from build123d import *

# Parameters (mm, degrees)
REVOLVE1_ANGLE = 270


with BuildPart() as part:
    # Sketch1 → Revolve1 (revolve)
    with BuildSketch(Plane.XY):
        with BuildLine():
            Line((0, 167.582815348), (0, 163))
            ThreePointArc((0, 163), (21.692969078, 161.550038974), (43, 157.225952056))
            Line((43, 157.225952056), (43, 87.225952056))
            Line((43, 87.225952056), (50, 87.225952056))
            Line((50, 87.225952056), (50, 57.225952056))
            Line((50, 57.225952056), (58, 57.225952056))
            Line((58, 57.225952056), (58, 112.225952056))
            Line((58, 112.225952056), (53, 112.225952056))
            Line((53, 112.225952056), (53, 117.225952056))
            Line((53, 117.225952056), (58, 117.225952056))
            Line((58, 117.225952056), (58, 122.225952056))
            Line((58, 122.225952056), (53, 122.225952056))
            Line((53, 122.225952056), (53, 127.225952056))
            Line((53, 127.225952056), (58, 127.225952056))
            Line((58, 127.225952056), (58, 132.225952056))
            Line((58, 132.225952056), (53, 132.225952056))
            Line((53, 132.225952056), (53, 137.225952056))
            Line((53, 137.225952056), (58, 137.225952056))
            Line((58, 137.225952056), (58, 142.225952056))
            Line((58, 142.225952056), (53, 142.225952056))
            Line((53, 142.225952056), (53, 147.225952056))
            Line((53, 147.225952056), (58, 147.225952056))
            Line((58, 147.225952056), (58, 157.225952056))
            ThreePointArc((58, 157.225952056), (29.458719495, 164.973282218), (0, 167.582815348))
        make_face()
    revolve(axis=Axis((0, 598.051491246, 0), (0, -1, 0)), revolution_arc=REVOLVE1_ANGLE)


solid = part.part
The listing builds one solid part. Answer for the finished solid, in the listing's coordinates (mm). A direction names the side the tool comes from. Coordinates: 2 decimals unless noted, no trailing zeros. Write each loop counter-clockwise with the first axis right and the second up, starting at its lowest first coordinate (ties: lowest second). Pieces come first, ordered by that corner, then holes. Notation, with made-up numbers: M -31,-1.5 L -15,-1.5 A10 cw -15,16.5 Z; hole C 73.25,59 d11. An arc over 180 degrees is marked long. Write each question's results on one line, items separated by ' | '.
Item 1: Given P1, Ø1, axis at y = 83.5, z = -37.5, coming from the +X side; P2, Ø8, axis at x = 4.5, z = 40, coming from the -Y side; P3, Ø5, axis at y = 82.5, z = -41.5, coming from the +X side, each flat-ended and moving along its own axis, determine where each tip first touches the part or whether it passes through.
Answer below:
P1: x = -32.5 | P2: y = 87.23 | P3: x = -23.75
Item 2: The part is cut by section C-C on z = -10. Determine the outline of the cut face in (x, y), and give its area (3 significant figures).
Answer below:
outline: M -57.13,57.23 L -48.99,57.23 L -48.99,87.23 L -41.82,87.23 L -41.82,157.23 A162.69 cw 0,162.69 L 0,167.28 A167.28 ccw -57.13,157.23 L -57.13,147.23 L -52.05,147.23 L -52.05,142.23 L -57.13,142.23 L -57.13,137.23 L -52.05,137.23 L -52.05,132.23 L -57.13,132.23 L -57.13,127.23 L -52.05,127.23 L -52.05,122.23 L -57.13,122.23 L -57.13,117.23 L -52.05,117.23 L -52.05,112.23 L -57.13,112.23 Z | area: 1,450 mm2
Item 3: For a pull along Z with two mould halves and no side action, classify faces 5 (the face through (-22, 87.226, 37.3)), 6 (the face through (-40, 130, 42)), 7 (the face through (46, 121, 0)) as released by +Z, released by -Z, zero draft, split by the parting line, or undercut.
Answer below:
face 5: undercut | face 6: split by the parting line | face 7: released by -Z
Item 4: The part is cut by section B-B on x = 5.5. Determine the outline of the cut face in (y, z), and give its area (3 significant figures).
Answer below:
outline: M 57.23,49.7 L 87.23,49.7 L 87.23,42.65 L 157.23,42.65 A162.91 cw 162.91,0 L 167.49,0 A167.49 ccw 157.23,57.74 L 147.23,57.74 L 147.23,52.71 L 142.23,52.71 L 142.23,57.74 L 137.23,57.74 L 137.23,52.71 L 132.23,52.71 L 132.23,57.74 L 127.23,57.74 L 127.23,52.71 L 122.23,52.71 L 122.23,57.74 L 117.23,57.74 L 117.23,52.71 L 112.23,52.71 L 112.23,57.74 L 57.23,57.74 Z | area: 1,430 mm2
Item 5: The part is cut by section A-A on y = 140. Determine the outline of the cut face in (x, z), and give its area (3 significant figures).
Answer below:
outline: M 0,-58 L 0,-43 A43 cw long 43,0 L 58,0 A58 ccw long Z | area: 3,570 mm2
Item 6: Consider probe 1 along Z at (x, y) = (-10.5, 118.5); probe 2 along X at (y, z) = (77.5, 3.5); probe 3 along Z at (x, y) = (45, 97). Determine where each line is inside the solid, lowest interval first. Write a range as [from, to].
Answer below:
probe 1: [-57.04, -41.7], [41.7, 57.04] | probe 2: [-57.89, -49.88], [49.88, 57.89] | probe 3: [0, 36.59]
Item 7: Which of the six approach directions +Z, -Z, +X, -X, +Y, -Y give full straight-line access (tool end or side, diameter ignored) to faces 1 (the face through (0, 121, -46)), 2 (the face through (-47, 127.226, 26)), 3 (the face through (-40, 140, 42)), 4 (the face through (-34.17, 72.02, 36.5))?
Answer below:
face 1: -Z, +X, +Y, -Y | face 2: none | face 3: +Y, -Y | face 4: -Y
